Geometry: see drawing. Coordinates: mm, zero at the bounding-box minimum. Coordinates: 2 decimals unless noted, no trailing zeros. Write each loop counter-clockwise with the first axis right and the second up, starting at its lowest first coordinate (ties: lowest second). Pieces come first, ordered by that corner, then holes. Notation, with made-up numbers: (16, 62.25) - (23, 62.25) arc R30 ccw to (23, 93.25) - close; hole circle Ø11 at (-1, 56.25). An arc over 180 degrees is marked (long way). One line per question, with ' | ' between items. Start each with the question number.
Q1. Cut plane A-A, the plane z = 7.25. Give the number of separate pieces and of enclosed holes in the cut face, plus the area to 4 significant figures.
Q2. Line query: line 1 (X direction, y = 21, z = 11.25) (1 decimal); line 2 (Y direction, x = 52, z = 6.5); line 3 (X direction, y = 30.5, z = 6.5). Output: solid intervals per line, ascending.
Q3. Cut plane B-B, the plane y = 24. Return loops of the section in (x, z), plus the area to 3 significant figures.
Q4. Draft query along X for the marked faces 1, 2, 3 and 4. Return one class per face: +X half, -X half, draft (parallel to the pull), parting line (faces both ways), or undercut.
Q5. Contact query for a flat-ended pin moving along its axis: P1, Ø5, axis at x = 37, z = 9.5, coming from the +Y side. Output: stop coordinate, or through.
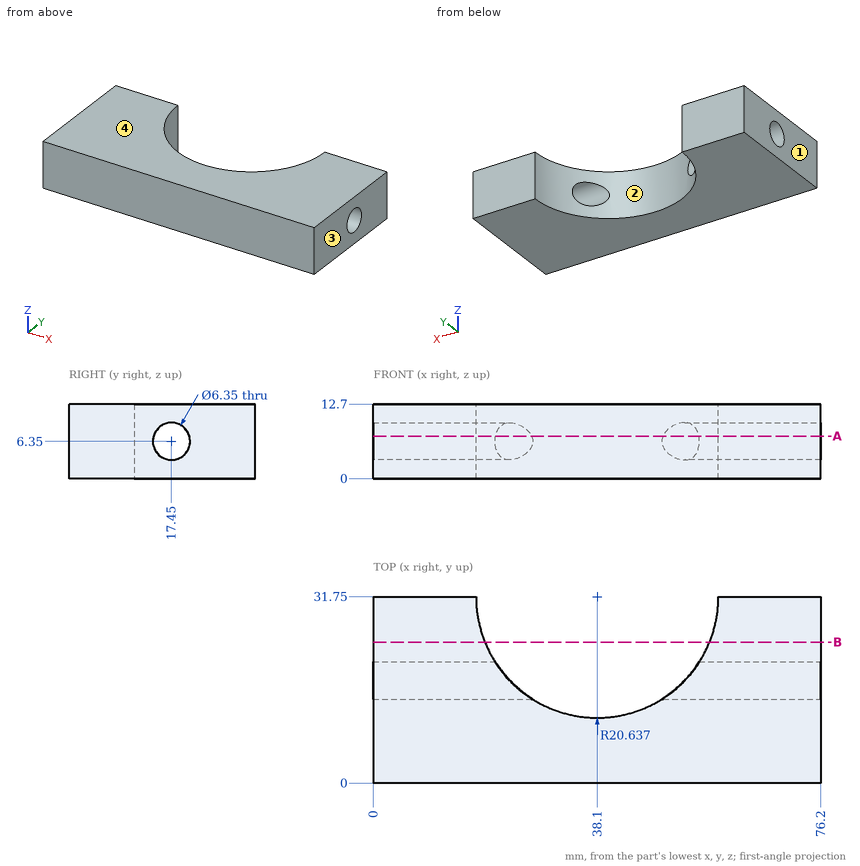
Reply:
1) separate pieces: 3 | enclosed holes: 0 | area: 1,465 mm^2
2) line 1: x = 0 to 20.5, 55.7 to 76.2 | line 2: y = 0 to 14.28 | line 3: x = 0 to 17.5, 58.7 to 76.2
3) outline: (0, 0) - (18.97, 0) - (18.97, 12.7) - (0, 12.7) - close; (57.23, 0) - (76.2, 0) - (76.2, 12.7) - (57.23, 12.7) - close | area: 482 mm^2
4) face 1: -X half | face 2: undercut | face 3: +X half | face 4: draft
5) P1: stops at y = 11.43
